Check sheet for the modelled part. Datum: model origin and axes. Units: mm. A direction names the side the tool comes from. Round coordinates to 2 decimals unless told otherwise and drop trailing zeros. Write each loop counter-clockwise with the first axis right and the second up, starting at its lowest first coordinate (ties: lowest second). Pieces come first, ordered by that corner, then holes.
Item 1: Cross-section at C-C on z = 255.5. Enter the section's corners in (x, y).
Item 2: Tool access check on faces 5 (the flat face through (0, -14, 520)), 6 (the flat face through (0, -13, 272)). Record the directions out of +Z, -Z, +X, -X, +Y, -Y that give a thin tool (end or side, any length) a straight path to the whole face; none if there is none.
Item 3: Material ranges on line 1 (Y direction, x = -3.25, z = 250); line 2 (Y direction, x = 11.5, z = 383), recorded low to high.
Item 4: Go/stop test with a flat-tipped pin: pin 1 Ø10 at (x, y) = (4.5, -3.5) entering from +Z. Record where the tip stops, or that it passes through.
Item 5: Cross-section at A-A on x = 0.25. Enter the section's corners in (y, z).
Item 6: Release check for a two-part mould opening along X. For faces 1 (the flat face through (0, 15, 272)), 2 (the flat face through (-15, 0, 272)), 3 (the flat face through (15, 0, 272)), 4 (the flat face through (-13, 0, 272)) record: +X half, -X half, draft (parallel to the pull), parting line (faces both ways), or undercut.
Autodesk Inventor part; units mm, degrees
ref_plane "Plano inicial" through (0, 0, 30) normal (0, 0, 1) x (1, 0, 0)
ref_plane "Plano final" through (0, 0, 520.0001) normal (0, 0, 1) x (1, 0, 0)
ref_plane "Plano de trabalho4" through (11, 160, 520) normal (0, 0, 1) x (1, 0, 0)
ref_plane "Plano inicial" through (0, 0, 30) normal (0, 0, 1) x (1, 0, 0)
ref_plane "Plano final" through (0, 0, 520.0001) normal (0, 0, 1) x (1, 0, 0)
sketch "Esboço" plane through (0, 0, 0) normal (0, 0, 1) x (1, 0, 0)
  line L0 (-15, -11) -> (-15, 11)
  line L1 (-11, 15) -> (11, 15)
  line L2 (15, 11) -> (15, -11)
  line L3 (11, -15) -> (-11, -15)
  arc A0 (-15, -11) -> (-11, -15) centre (-11, -11) ccw
  arc A1 (15, 11) -> (11, 15) centre (11, 11) ccw
  arc A2 (-11, 15) -> (-15, 11) centre (-11, 11) ccw
  arc A3 (11, -15) -> (15, -11) centre (11, -11) ccw
  arc A4 (-11, 13) -> (-13, 11) centre (-11, 11) ccw
  line L4 (-11, 13) -> (11, 13)
  arc A5 (13, 11) -> (11, 13) centre (11, 11) ccw
  line L5 (13, 11) -> (13, -11)
  arc A6 (11, -13) -> (13, -11) centre (11, -11) ccw
  line L6 (11, -13) -> (-11, -13)
  arc A7 (-13, -11) -> (-11, -13) centre (-11, -11) ccw
  line L7 (-13, -11) -> (-13, 11)
  line L8 (0, 22.1598) -> (0, -22.1598) construction
  line L9 (-22.1598, 0) -> (22.1598, 0) construction
  dimension "d7" = 4
  dimension "d9" = 30
  dimension "d11" = 30
  dimension "d12" = 2
  dimension "d15" = 15
  dimension "d16" = 15
extrude "Corpo" add sketch "Esboço" along normal up to surface (490.0001 mm away) from surface at 30
sketch "Sketch3" plane through (0, 0, 0) normal (0, 0, 1) x (1, 0, 0)
  line L0 (0, 0) -> (10, 0)
ref_plane "Work Plane3" through (0, 0, 0) normal (0, -1, 0) x (1, 0, 0)
sketch "Sketch4" plane through (0, 0, 0) normal (0, -1, 0) x (1, 0, 0)
  line L0 (-2, 30) -> (12, 30)
  line L1 (-2, 520.0001) -> (12, 520.0001)
  dimension "d18" = 490.0001
ref_plane "Plano de trabalho4" through (11, 160, 520) normal (0, 0, 1) x (1, 0, 0)
split "Dividir1" plane through (11, 160, 520) removes the side toward (0, 0, 1)
ref_plane "Plano de trabalho5" through (11, -290, 30) normal (0, 0, -1) x (-1, 0, 0)
split "Dividir2" plane through (11, -290, 30) removes the side toward (0, 0, -1)
equation "\"d7\" = G_IR"
equation "\"d9\" = G_W"
equation "\"d11\" = G_H"
equation "\"d12\" = G_T"
equation "\"d15\" = 0.5 * d9"
equation "\"d16\" = 0.5 * d11"
equation "\"d3\" = G_L"
equation "\"G_W\" = 30"
equation "\"G_H\" = 30"
equation "\"G_T\" = 2"
equation "\"G_IR\" = 4"
equation "\"G_L\" = d18"
equation "\"G_OFFSET_END\" = -29.99991"
equation "\"d14\" = G_OFFSET_END + B_L"
properties part number "ISO 10799-2 - 30x30x2 - 490" material "Aço, suave"
Response values:
1. outline: (-15, -11) arc R4 ccw to (-11, -15) - (11, -15) arc R4 ccw to (15, -11) - (15, 11) arc R4 ccw to (11, 15) - (-11, 15) arc R4 ccw to (-15, 11) - close; hole (-13, -11) arc R2 ccw to (-11, -13) - (11, -13) arc R2 ccw to (13, -11) - (13, 11) arc R2 ccw to (11, 13) - (-11, 13) arc R2 ccw to (-13, 11) - close
2. face 5: +Z, +X, -X, +Y, -Y
2. face 6: +Z, -Z
3. line 1: y = -15 to -13, 13 to 15
3. line 2: y = -14.97 to -12.94, 12.94 to 14.97
4. pin 1: passes through
5. outline: (-15, 30) - (-13, 30) - (-13, 520) - (-15, 520) - close; (13, 30) - (15, 30) - (15, 520) - (13, 520) - close
6. face 1: draft
6. face 2: -X half
6. face 3: +X half
6. face 4: undercut
